Geometry: final body of the model. Coordinates: model frame, mm. A direction names the side the tool comes from. Round coordinates to 2 decimals unless told otherwise and drop trailing zeros. Loops run counter-clockwise (first coordinate to the right, second up) from the corner with the lowest first, then second, coordinate; pieces in that order, holes last. Notation, with made-up numbers: M -15,20 L 28,20 A12 cw 28,39 Z; hole C 29.25,26 d5. An arc over 180 degrees is marked long. Answer as a JSON object with one key per item and string values.
```python
from build123d import *

# Parameters (mm, degrees)
SKETCH_3_R          = 1.55
SKETCH_3_R_2        = 3.375
EXTRUDE_1_DEPTH     = 4.5
FILLET_1_R          = 5
CUT_EXTRUDE_2_REACH = 200.281
FILLET_3_R          = 3
EXTRUDE_5096_DEPTH  = 4.5


with BuildPart() as part:
    # 草图3 → 凸台-拉伸1 (new body)
    with BuildSketch(Plane(origin=(0, 0, 0), x_dir=(1, 0, 0), z_dir=(0, 1, 0))):
        with BuildLine():
            Line((94.694386062, -62.928175745), (41.131907973, -24.012757507))
            ThreePointArc((41.131907973, -24.012757507), (34.497097301, -25.063608282), (35.547948076, -31.698418954))
            Line((35.547948076, -31.698418954), (84.136405992, -67))
            Line((84.136405992, -67), (77.5, -67))
            Line((77.5, -67), (77.5, -69))
            Line((77.5, -69), (75, -69))
            Line((75, -69), (75, -70.45))
            Line((75, -70.45), (78.5, -70.45))
            Line((78.5, -70.45), (78.5, -68.25))
            Line((78.5, -68.25), (81.75, -68.25))
            Line((81.75, -68.25), (81.75, -70.45))
            Line((81.75, -70.45), (83.75, -70.45))
            Line((83.75, -70.45), (83.75, -73.55))
            Line((83.75, -73.55), (81.75, -73.55))
            Line((81.75, -73.55), (81.75, -75.75))
            Line((81.75, -75.75), (78.5, -75.75))
            Line((78.5, -75.75), (78.5, -73.55))
            Line((78.5, -73.55), (75, -73.55))
            Line((75, -73.55), (75, -75))
            Line((75, -75), (77.5, -75))
            Line((77.5, -75), (77.5, -77))
            Line((77.5, -77), (84.136405992, -77))
            Line((84.136405992, -77), (84.470607294, -77))
            Line((84.470607294, -77), (83.673412582, -78.097244389))
            Line((83.673412582, -78.097244389), (94.999650503, -86.326237921))
            Line((94.999650503, -86.326237921), (41.671203749, -139.654684675))
            Line((41.671203749, -139.654684675), (30.676078989, -140.941956792))
            ThreePointArc((30.676078989, -140.941956792), (30.043220441, -145.236869059), (29.290205532, -149.512351472))
            ThreePointArc((29.290205532, -149.512351472), (29.56084749, -151.429597804), (30.946340523, -152.782184076))
            Line((30.946340523, -152.782184076), (40.152805518, -157.170406668))
            Line((40.152805518, -157.170406668), (46.916516286, -146.430187419))
            Line((46.916516286, -146.430187419), (101.962013194, -91.384690511))
            Line((101.962013194, -91.384690511), (106.325888424, -94.555231453))
            Line((106.325888424, -94.555231453), (122.783875489, -71.902755611))
            Line((122.783875489, -71.902755611), (100.131399646, -55.444768547))
            Line((100.131399646, -55.444768547), (94.694386062, -62.928175745))
        make_face()
        with Locations(Location((39.335, -149.432300402, 0), (0, 0, 270))):
            Circle(SKETCH_3_R, mode=Mode.SUBTRACT)
        with Locations(Location((44.044221455, -32, 0), (0, 0, 270))):
            Circle(SKETCH_3_R, mode=Mode.SUBTRACT)
        with Locations(Location((60.224561343, -43.755705046, 0), (0, 0, 270))):
            Circle(SKETCH_3_R, mode=Mode.SUBTRACT)
        with BuildLine():
            ThreePointArc((95.08466389, -74.720558792), (96.858054238, -76.0090023), (95.569610731, -77.782392648))
            Line((95.569610731, -77.782392648), (93.841156135, -78.056152962))
            ThreePointArc((93.841156135, -78.056152962), (92.067765787, -76.767709455), (93.356209294, -74.994319106))
            Line((93.356209294, -74.994319106), (95.08466389, -74.720558792))
        make_face(mode=Mode.SUBTRACT)
        with BuildLine():
            Line((103.222963142, -84.872434742), (102.949202828, -83.143980146))
            ThreePointArc((102.949202828, -83.143980146), (104.237646335, -81.370589797), (106.011036684, -82.659033304))
            Line((106.011036684, -82.659033304), (106.284796997, -84.3874879))
            ThreePointArc((106.284796997, -84.3874879), (104.99635349, -86.160878249), (103.222963142, -84.872434742))
        make_face(mode=Mode.SUBTRACT)
        with Locations(Location((103.228644035, -75, 0), (0, 0, 270))):
            Circle(SKETCH_3_R_2, mode=Mode.SUBTRACT)
        with BuildLine():
            ThreePointArc((111.372624181, -75.279441208), (109.599233832, -73.9909977), (110.887677339, -72.217607352))
            Line((110.887677339, -72.217607352), (112.616131935, -71.943847038))
            ThreePointArc((112.616131935, -71.943847038), (114.389522284, -73.232290545), (113.101078777, -75.005680894))
            Line((113.101078777, -75.005680894), (111.372624181, -75.279441208))
        make_face(mode=Mode.SUBTRACT)
        with BuildLine():
            Line((103.234324929, -65.127565258), (103.508085243, -66.856019854))
            ThreePointArc((103.508085243, -66.856019854), (102.219641736, -68.629410203), (100.446251387, -67.340966696))
            Line((100.446251387, -67.340966696), (100.172491073, -65.6125121))
            ThreePointArc((100.172491073, -65.6125121), (101.46093458, -63.839121751), (103.234324929, -65.127565258))
        make_face(mode=Mode.SUBTRACT)
    extrude(amount=EXTRUDE_1_DEPTH)

    # 圆角-美观1
    fillet_1_edges = [part.edges().sort_by_distance(p)[0] for p in [
        (100.131399646, 2.25, 55.444768547),
        (122.783875489, 2.25, 71.902755611),
    ]]
    fillet(fillet_1_edges, radius=FILLET_1_R)

    # 草图4 → 圆弧-美观2 (cut, up to next)
    with BuildSketch(Plane(origin=(0, 4.5, 0), x_dir=(1, 0, 0), z_dir=(0, 1, 0)), mode=Mode.PRIVATE) as cut_extrude_2_sk1:
        with BuildLine():
            ThreePointArc((118.738790517, -68.963829349), (109.994899962, -65.687047674), (104.176484618, -58.383694808))
            Line((104.176484618, -58.383694808), (118.738790517, -68.963829349))
        make_face()
    cut_extrude_2_tool1 = extrude(cut_extrude_2_sk1.sketch, amount=-CUT_EXTRUDE_2_REACH, mode=Mode.PRIVATE) & part.part
    # 草图4 → 圆弧-美观2 (cut, up to next)
    with BuildSketch(Plane(origin=(0, 4.5, 0), x_dir=(1, 0, 0), z_dir=(0, 1, 0)), mode=Mode.PRIVATE) as cut_extrude_2_sk2:
        with BuildLine():
            Line((119.844949227, -75.947840583), (109.264814686, -90.510146481))
            ThreePointArc((109.264814686, -90.510146481), (112.204348353, -81.521230905), (119.844949227, -75.947840583))
        make_face()
    cut_extrude_2_tool2 = extrude(cut_extrude_2_sk2.sketch, amount=-CUT_EXTRUDE_2_REACH, mode=Mode.PRIVATE) & part.part
    add(cut_extrude_2_tool1.solids().sort_by_distance((110.868828, 4.5, 64.48419))[0], mode=Mode.SUBTRACT)
    add(cut_extrude_2_tool2.solids().sort_by_distance((113.606622, 4.5, 82.540042))[0], mode=Mode.SUBTRACT)

    # 圆角-美观3
    fillet_3_edges = [part.edges().sort_by_distance(p)[0] for p in [
        (94.999650503, 2.25, 86.326237921),
        (94.694386062, 2.25, 62.928175745),
        (106.325888424, 2.25, 94.555231453),
        (40.152805518, 2.25, 157.170406668),
        (118.738790517, 2.25, 68.963829349),
        (104.176484618, 2.25, 58.383694808),
        (119.844949227, 2.25, 75.947840583),
        (109.264814686, 2.25, 90.510146481),
    ]]
    fillet(fillet_3_edges, radius=FILLET_3_R)

    # 草图5 → Extrude 5096 (add)
    with BuildSketch(Plane(origin=(0, 0, 0), x_dir=(1, 0, 0), z_dir=(0, 1, 0))):
        with BuildLine():
            Line((41.131907973, -24.012757507), (54.395000648, -33.648958388))
            ThreePointArc((54.395000648, -33.648958388), (47.749518962, -27.625359459), (42.549937685, -20.317108954))
            ThreePointArc((42.549937685, -20.317108954), (39.186571182, -12.543642943), (37.467706796, -4.25))
            Line((37.467706796, -4.25), (30.5, -4.25))
            Line((30.5, -4.25), (30.5, -3.25))
            Line((30.5, -3.25), (30.5, 2.25))
            Line((30.5, 2.25), (26.902552576, 2.25))
            ThreePointArc((26.902552576, 2.25), (27.35989158, -8.024554542), (29.428853503, -18.099028552))
            ThreePointArc((29.428853503, -18.099028552), (29.710927986, -19.386919832), (29.821122157, -20.700726214))
            ThreePointArc((29.821122157, -20.700726214), (31.390100135, -26.873623403), (35.547948076, -31.698418954))
            Line((35.547948076, -31.698418954), (41.131907973, -24.012757507))
        make_face()
    extrude(amount=EXTRUDE_5096_DEPTH)


solid = part.part
```
1) Cut plane C-C on y = 3.15. Count the separate pieces of the cut face and the enclosed holes in it, and give its area (3 significant figures).
Geometry results:
{"separate pieces": "1", "enclosed holes": "8", "area": "2,470 mm2"}
2) Cut plane B-B on x = 34. Return the cut outline in (y, z), and give its area (3 significant figures).
Geometry results:
{"outline": "M 0,4.25 L 4.5,4.25 L 4.5,30.39 L 0,30.39 Z; M 0,140.55 L 4.5,140.55 L 4.5,154.24 L 0,154.24 Z", "area": "179 mm2"}
3) Cut plane A-A on x = 66. Return the cut outline in (y, z).
Geometry results:
{"outline": "M 0,42.08 L 4.5,42.08 L 4.5,53.82 L 0,53.82 Z; M 0,115.33 L 4.5,115.33 L 4.5,127.35 L 0,127.35 Z"}
4) Cut plane D-D on z = 52. Return the cut outline in (x, y).
Geometry results:
{"outline": "M 63.49,0 L 79.65,0 L 79.65,4.5 L 63.49,4.5 Z"}
5) Pull-direction query (X, two-part tool) for faces 1 (the face through (104.204, 2.218, 81.376)), 2 (the face through (29, 2, -2.25)), 3 (the face through (30.053, 2.218, 145.177)); classes: +X half, -X half, draft (parallel to the pull), parting line (faces both ways), or undercut.
Geometry results:
{"face 1": "undercut", "face 2": "draft", "face 3": "-X half"}
6) Set-up query: faces 4 (the face through (83.75, 2, 72)), 5 (the face through (34, 2, 4.25)), 6 (the face through (99.655, 2.282, 57.686)). Return all of +Z, -Z, +X, -X, +Y, -Y with unobstructed straight access to the full face (end or side cutting, diameter ignored); none if empty.
Geometry results:
{"face 4": "-X, +Y, -Y", "face 5": "-Z, +X, +Y, -Y", "face 6": "-Z, +Y, -Y"}
7) Line query: probe 1 along Z at (x, y) = (43.5, 1.3); probe 2 along Z at (x, y) = (44, 2.2); probe 3 along Z at (x, y) = (48.5, 2.8). Output: solid intervals per line, ascending.
Geometry results:
{"probe 1": "21.93 to 30.55, 33.45 to 37.48, 137.83 to 151.86", "probe 2": "22.71 to 30.45, 33.55 to 37.84, 137.33 to 151.06", "probe 3": "28.45 to 41.11, 132.83 to 144.85"}
8) First-contact query: pin 1 (2 mm diameter, centred on y = 3.5, z = 44.5, fed in from -X); pin 2 (0.9 mm diameter, centred on y = 2.5, z = 71.5, fed in from -X); pin 3 (1.8 mm diameter, centred on x = 76, y = 2, fed in from -Z). Flat tips, straight axial feed; report the tip coordinate or a pass-through.
Geometry results:
{"pin 1": "x = 51.79", "pin 2": "x = 83.75", "pin 3": "z = 48.69"}
